```python
from build123d import *

# Parameters (mm, degrees)
F2_DEPTH  = 12.7
F3_R      = 12.7
F4_R      = 19.05
F5_R      = 8.88999
F6_R      = 2.53999
F7_R      = 1.27
F8_R      = 2.2225
F9_DEPTH  = 6.35
F10_R     = 1.651
F11_DEPTH = 9.525
F13_DEPTH = 1.27


# Not quite as in the source:
# - a fillet or chamfer is up to 0.001 mm smaller than in the source, because OpenCascade refuses the exact size


with BuildPart() as f2:
    # F1 (on Right) → F2 (new body)
    with BuildSketch(Plane.YZ):
        Polygon((-26.67, -19.05), (-26.67, 0), (-25.4, 1.27), (-25.4, 12.7), (-33.02, 12.7), (-33.02, -25.4), (-11.43, -25.4), (-11.43, -38.1), (-5.08, -38.1), (-5.08, -19.05), align=None)
    extrude(amount=F2_DEPTH)

    # F3
    f3_edges = [f2.edges().sort_by_distance(p)[0] for p in [
        (6.35, -26.67, -19.05),
    ]]
    fillet(f3_edges, radius=F3_R)

    # F4
    f4_edges = [f2.edges().sort_by_distance(p)[0] for p in [
        (6.35, -33.02, -25.4),
    ]]
    fillet(f4_edges, radius=F4_R)

    # F5 (radius 8.89 in the source; OpenCascade refuses exactly that, so slightly less here)
    f5_edges = [f2.edges().sort_by_distance(p)[0] for p in [
        (6.35, -5.08, -19.05),
    ]]
    fillet(f5_edges, radius=F5_R)

    # F6 (radius 2.54 in the source; OpenCascade refuses exactly that, so slightly less here)
    f6_edges = [f2.edges().sort_by_distance(p)[0] for p in [
        (6.35, -11.43, -25.4),
    ]]
    fillet(f6_edges, radius=F6_R)

    # F7
    f7_edges = [f2.edges().sort_by_distance(p)[0] for p in [
        (6.35, -26.67, 0),
        (6.35, -25.4, 1.27),
        (6.35, -25.4, 12.7),
        (6.35, -33.02, 12.7),
        (6.35, -11.43, -38.1),
        (6.35, -5.08, -38.1),
    ]]
    fillet(f7_edges, radius=F7_R)

    # F8 (on face) → F9 (cut)
    with BuildSketch(Plane.XZ.offset(11.43)):
        with Locations((6.35, -32.385)):
            Circle(F8_R)
    extrude(amount=-F9_DEPTH, mode=Mode.SUBTRACT)

    # F10 (on face) → F11 (join)
    with BuildSketch(Plane(origin=(0, 0, 0), x_dir=(0, -1, 0), z_dir=(-1, 0, 0))):
        with Locations((29.21, 8.89)):
            Circle(F10_R)
    extrude(amount=F11_DEPTH)

    # F12 (on face) → F13 (join)
    with BuildSketch(Plane(origin=(0, 0, 0), x_dir=(0, -1, 0), z_dir=(-1, 0, 0))):
        with BuildLine():
            Line((31.75, -6.35), (33.02, -6.35))
            Line((33.02, -6.35), (33.02, 11.43))
            ThreePointArc((33.02, 11.43), (32.6480256121, 12.3280256121), (31.75, 12.7))
            Line((31.75, 12.7), (31.75, -6.35))
        make_face()
    extrude(amount=F13_DEPTH)


solid = f2.part
```
Work out the finished part from the listing and answer in its coordinate system (mm). A direction names the side the tool comes from. Coordinates: 2 decimals unless noted, no trailing zeros. Order: outer loops, then holes, each group sorted by start corner. A loop starts at its lowest first (then second) coordinate and runs counter-clockwise, first axis right, second up. Notation, with made-up numbers: (18.5, 3) - (53.5, 3) arc R19 ccw to (53.5, 34) - close; hole circle Ø11 at (71, 50). An arc over 180 degrees is marked (long way). Answer as a JSON object with one key per item and string values.
1. The mould has two halves that part along Z. Classify faces 6 (the face through (6, -26.67, -3)), 7 (the face through (6.439, -12.154, -26.164)), 8 (the face through (6.439, -25.782, 12.338)): +Z half, -Z half, draft (parallel to the pull), parting line (faces both ways), or undercut.
Output values:
{"face 6": "undercut", "face 7": "-Z half", "face 8": "+Z half"}
2. Consider line 1 (Y direction, x = 9.75, z = 9); line 2 (Z direction, x = 6.35, y = -9.5); line 3 (X direction, y = -7.75, z = -27.5). Determine where each line is inside the solid, lowest interval first.
Output values:
{"line 1": "y = -33.02 to -25.4", "line 2": "z = -38.1 to -34.61, -30.16 to -20.26", "line 3": "x = 0 to 12.7"}
3. Find section D-D on y = -29.21. Determine the outline of the cut face in (x, z) (3 decimals), plus the area to 3 significant figures.
Output values:
{"outline": "(-9.525, 7.239) - (0, 7.239) - (0, -17.78) - (12.7, -17.78) - (12.7, 12.7) - (0, 12.7) - (0, 10.541) - (-9.525, 10.541) - close", "area": "419 mm²"}
4. Each of these flat-tipped pins is pushed along its axis until it touches: P1, Ø10, axis at y = -23, z = -5.5, coming from the -X side; P2, Ø1, axis at y = -32.5, z = 5.5, coming from the -X side; P3, Ø5, axis at x = 5, z = 7, coming from the +Y side. Where does it stop, or does it pass through?
Output values:
{"P1": "stops at x = 0", "P2": "stops at x = -1.27", "P3": "stops at y = -25.4"}
5. A tool of negligible diameter and unlimited length cuts with its end or side. For faces 1 (the face through (-1, -31.75, 3)), 2 (the face through (-4.696, -29.972, 7.425)), 3 (the face through (4.8, -11.43, -34.3)), 4 (the face through (-1.27, -32, 3)), 5 (the face through (6.44, -23.05, -15.23)), from which of +Z, -Z, +X, -X, +Y, -Y can it reach the whole face along a straight path? Write none if from no direction.
Output values:
{"face 1": "+Z, -Z, -X", "face 2": "-X", "face 3": "-Z, +X, -X, -Y", "face 4": "+Z, -Z, -X, -Y", "face 5": "+X, -X, +Y"}
6. Find section B-B on z = 8.89. Determine the outline of the cut face in (x, y) (3 decimals).
Output values:
{"outline": "(-9.525, -30.861) - (0, -30.861) - (0, -31.75) - (-1.27, -31.75) - (-1.27, -33.02) - (12.7, -33.02) - (12.7, -25.4) - (0, -25.4) - (0, -27.559) - (-9.525, -27.559) - close"}
